Check sheet for the modelled part. Datum: model origin and axes. Units: mm. Round coordinates to 2 decimals unless told otherwise and drop trailing zeros. Loops run counter-clockwise (first coordinate to the right, second up) from the corner with the lowest first, then second, coordinate; pieces in that order, holes last. Notation, with made-up numbers: (26.25, 75.5) - (65.25, 75.5) arc R21 ccw to (65.25, 90.5) - close; hole circle Ø5 at (-7.75, 14). An arc over 180 degrees is marked (long way). Return JSON: item names as keys, results as strings.
Autodesk Inventor part; units mm, degrees
ref_plane "YZ Plane" through (0, 0, 0) normal (1, 0, 0) x (0, 1, 0)
ref_plane "XZ Plane" through (0, 0, 0) normal (0, 1, 0) x (-1, 0, 0)
ref_plane "XY Plane" through (0, 0, 0) normal (0, 0, 1) x (1, 0, 0)
sketch "スケッチ1" plane through (0, 0, 0) normal (0, 0, 1) x (1, 0, 0)
  line L0 (0, 3.1754) -> (2.75, 1.5877)
  line L1 (2.75, 1.5877) -> (2.75, -1.5877)
  line L2 (2.75, -1.5877) -> (0, -3.1754)
  line L3 (0, -3.1754) -> (-2.75, -1.5877)
  line L4 (-2.75, -1.5877) -> (-2.75, 1.5877)
  line L5 (-2.75, 1.5877) -> (0, 3.1754)
  point P0 (0, 0)
  point P1 (0, 0)
  dimension "d0" = 5.5
extrude "押し出し1" add sketch "スケッチ1" along normal blind 70
sketch "スケッチ2" plane through (0, 0, 70) normal (0, 0, 1) x (1, 0, 0)
  point P0 (0, 0)
hole "穴1" at (0, 0, 70) direction (0, 0, -1) diameter 2.459 depth 8.8 tip angle 118
sketch "スケッチ3" plane through (0, 0, 0) normal (0, 0, -1) x (-1, 0, 0)
  point P0 (0, 0)
hole "穴2" at (0, 0, 0) direction (0, 0, 1) diameter 2.459 depth 8.8 tip angle 118
properties part number "アルミスペーサー(六角・酸洗処理）_ASL-370E" material "アルミニウム 6061"
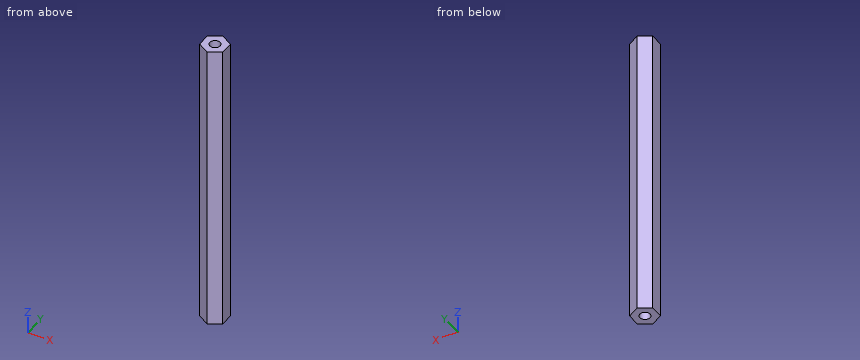
Q1. Scan lines: probe 1 along Y at (x, z) = (0, 4); probe 2 along X at (y, z) = (0, 5.75); probe 3 along Y at (x, z) = (-1.5, 28). Record each from-to range of solid material in increasing order. Write a range as [from, to].
Answer key:
{"probe 1": "y = [-3.18, -1.23], [1.23, 3.18]", "probe 2": "x = [-2.75, -1.23], [1.23, 2.75]", "probe 3": "y = [-2.31, 2.31]"}
Q2. Sectioned sample at B-B (y = -2.5). Enter the section's corners in (x, z).
Answer key:
{"outline": "(-1.17, 0) - (1.17, 0) - (1.17, 70) - (-1.17, 70) - close"}
Q3. Sectioned sample at A-A (z = 62). Enter the section's corners in (x, y).
Answer key:
{"outline": "(-2.75, -1.59) - (0, -3.18) - (2.75, -1.59) - (2.75, 1.59) - (0, 3.18) - (-2.75, 1.59) - close; hole circle Ø2.46 at (0, 0)"}
Q4. Depth check by flat-ended pin: P1, Ø2, axis at x = -0.5, z = 20.5, coming from the +Y side. Enter the tip coordinate at first touch or a pass-through.
Answer key:
{"P1": "stops at y = 3.18"}
